from build123d import *

# Parameters (mm, degrees)
F0_R     = 10
F0_W     = 22
F0_H     = 28
F0_R_2   = 6
F1_DEPTH = 2


with BuildPart() as f1:
    # F0 (on Top) → F1 (new body)
    with BuildSketch(Plane.XY):
        Polygon((0, 0), (146, 0), (146, 27.341935), (76, 27.341935), (76, 122.341935), (38, 122.341935), (0, 122.341935), align=None)
        with Locations((13, 27.341935)):
            Circle(F0_R, mode=Mode.SUBTRACT)
        with Locations((38, 27.341935)):
            Circle(F0_R, mode=Mode.SUBTRACT)
        with Locations((63, 27.341935)):
            Circle(F0_R, mode=Mode.SUBTRACT)
        with Locations((19, 67.341935)):
            Rectangle(F0_W, F0_H, mode=Mode.SUBTRACT)
        with Locations((57, 67.341935)):
            Circle(F0_R_2, mode=Mode.SUBTRACT)
    extrude(amount=F1_DEPTH)


solid = f1.part
Geometry: final body of the model. Coordinates: model frame, mm. Round coordinates to 2 decimals unless told otherwise and drop trailing zeros. Loops run counter-clockwise (first coordinate to the right, second up) from the corner with the lowest first, then second, coordinate; pieces in that order, holes last.
Q1. Material intervals for L1, parallel to Y at x = 38, z = 0.95; L2, parallel to X at y = 68, z = 1.6; L3, parallel to X at y = 36.5, z = 0.65, sorted ascending.
Q2. Section B-B on x = 13. Return loops of the section in (y, z).
Q3. Pull-direction query (X, two-part tool) for faces 1 (the cylindrical face through (10.83, 17.58, 0.99)), 2 (the flat face through (56, 48, 2)); classes: released by +X, released by -X, zero draft, split by the parting line, or undercut.
Q4. Section A-A on x = 38. Return loops of the section in (y, z).
Q5. Section C-C on y = 31. Return loops of the section in (x, z), plus the area to 3 significant figures.
Q6. Section D-D on z = 1.7. Return loops of the section in (x, y).
Q7. Pin query (flat end, axial travel): P1, Ø1, axis at x = 92.5, z = 0.5, coming from the +Y side; P2, Ø1, axis at y = 93, z = 1, coming from the +X side. Return the tip coordinate at first contact, or that it passes through.
Evaluation:
1. L1: y = 0 to 17.34, 37.34 to 122.34
1. L2: x = 0 to 8, 30 to 51.04, 62.96 to 76
1. L3: x = 0 to 8.98, 17.02 to 33.98, 42.02 to 58.98, 67.02 to 76
2. outline: (0, 0) - (17.34, 0) - (17.34, 2) - (0, 2) - close; (37.34, 0) - (53.34, 0) - (53.34, 2) - (37.34, 2) - close; (81.34, 0) - (122.34, 0) - (122.34, 2) - (81.34, 2) - close
3. face 1: undercut
3. face 2: zero draft
4. outline: (0, 0) - (17.34, 0) - (17.34, 2) - (0, 2) - close; (37.34, 0) - (122.34, 0) - (122.34, 2) - (37.34, 2) - close
5. outline: (0, 0) - (3.69, 0) - (3.69, 2) - (0, 2) - close; (22.31, 0) - (28.69, 0) - (28.69, 2) - (22.31, 2) - close; (47.31, 0) - (53.69, 0) - (53.69, 2) - (47.31, 2) - close; (72.31, 0) - (76, 0) - (76, 2) - (72.31, 2) - close
5. area: 40.3 mm2
6. outline: (0, 0) - (146, 0) - (146, 27.34) - (76, 27.34) - (76, 122.34) - (0, 122.34) - close; hole circle Ø20 at (13, 27.34); hole (8, 53.34) - (30, 53.34) - (30, 81.34) - (8, 81.34) - close; hole circle Ø20 at (38, 27.34); hole circle Ø12 at (57, 67.34); hole circle Ø20 at (63, 27.34)
7. P1: stops at y = 27.34
7. P2: stops at x = 76
